Geometry: see drawing. Coordinates: mm, zero at the bounding-box minimum. A direction names the side the tool comes from. Coordinates: 2 decimals unless noted, no trailing zeros. Write each loop counter-clockwise with the first axis right and the second up, starting at its lowest first coordinate (ties: lowest second). Pieces come first, ordered by that corner, then holes. Notation, with made-up numbers: M 74,44 L 114,44 A26 cw 114,82 Z; hole C 87.25,-35.5 d2. An arc over 180 degrees is marked long. One line per item, written item: value. Start each with the question number.
Item 1: Pin query (flat end, axial travel): P1, Ø6, axis at x = 47.5, z = 30, coming from the -Y side; P2, Ø5, axis at x = 15, z = 33, coming from the -Y side; P3, Ø10, axis at x = 28.5, y = 39, coming from the +Z side. Return the tip coordinate at first contact, or that it passes through.
Item 2: Cut plane D-D, the plane x = 56. Output: boundary loops of the cut face in (y, z).
Item 3: Cut plane C-C, the plane x = 35. Output: boundary loops of the cut face in (y, z).
Item 4: Set-up query: the marked faces 1 and 2. Return all of +Z, -Z, +X, -X, +Y, -Y with unobstructed straight access to the full face (end or side cutting, diameter ignored); none if empty.
Item 5: Ray query, L1, parallel to X at y = 36.5, z = 29; L2, parallel to Y at x = 65.5, z = 25; L3, parallel to X at y = 17, z = 44. Return the intervals inside material, ascending. Write a range as from..to.
Item 6: Cut plane A-A, the plane y = 25. Output: boundary loops of the cut face in (x, z).
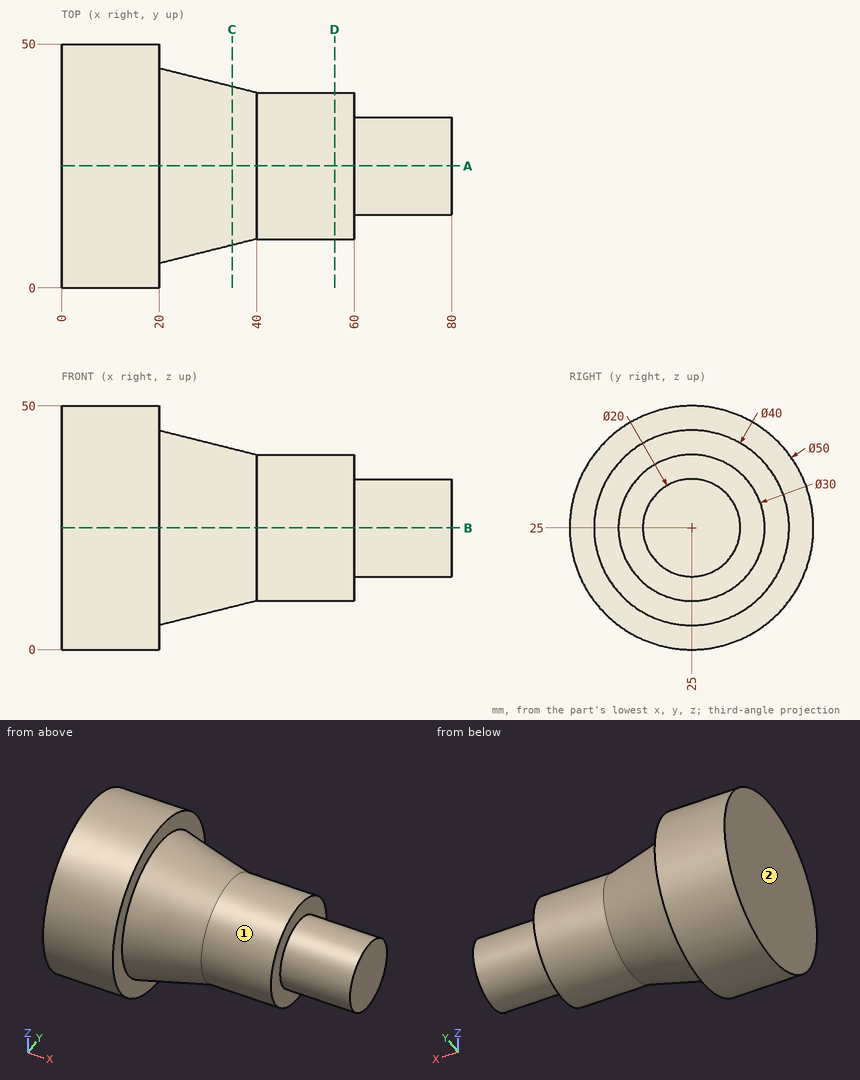
From the geometry:
1. P1: stops at y = 10.13
1. P2: stops at y = 0.61
1. P3: stops at z = 40.78
2. outline: C 25,25 d30
3. outline: C 25,25 d32.5
4. face 1: +X
4. face 2: +Z, -Z, -X, +Y, -Y
5. L1: x = 0..60
5. L2: y = 15..35
5. L3: x = 0..20
6. outline: M 0,0 L 20,0 L 20,5 L 40,10 L 60,10 L 60,15 L 80,15 L 80,35 L 60,35 L 60,40 L 40,40 L 20,45 L 20,50 L 0,50 Z
